The figure shows three views and two pictorial views of one solid part (mm, origin at its lowest corner). Answer the questions. A direction names the side the tool comes from. Coordinates: 2 decimals unless noted, no trailing zeros. Order: outer loops, then holes, each group sorted by start corner. A loop starts at its lowest first (then second) coordinate and runs counter-clockwise, first axis right, second up. Notation, with made-up numbers: (71.25, -31.5) -> (77.25, -31.5) arc R21 ccw to (77.25, -22.5) -> close; hole circle Ø5 at (4.5, 81.25). An arc over 180 degrees is marked (long way). Return JSON: item names as keys, results as strings.
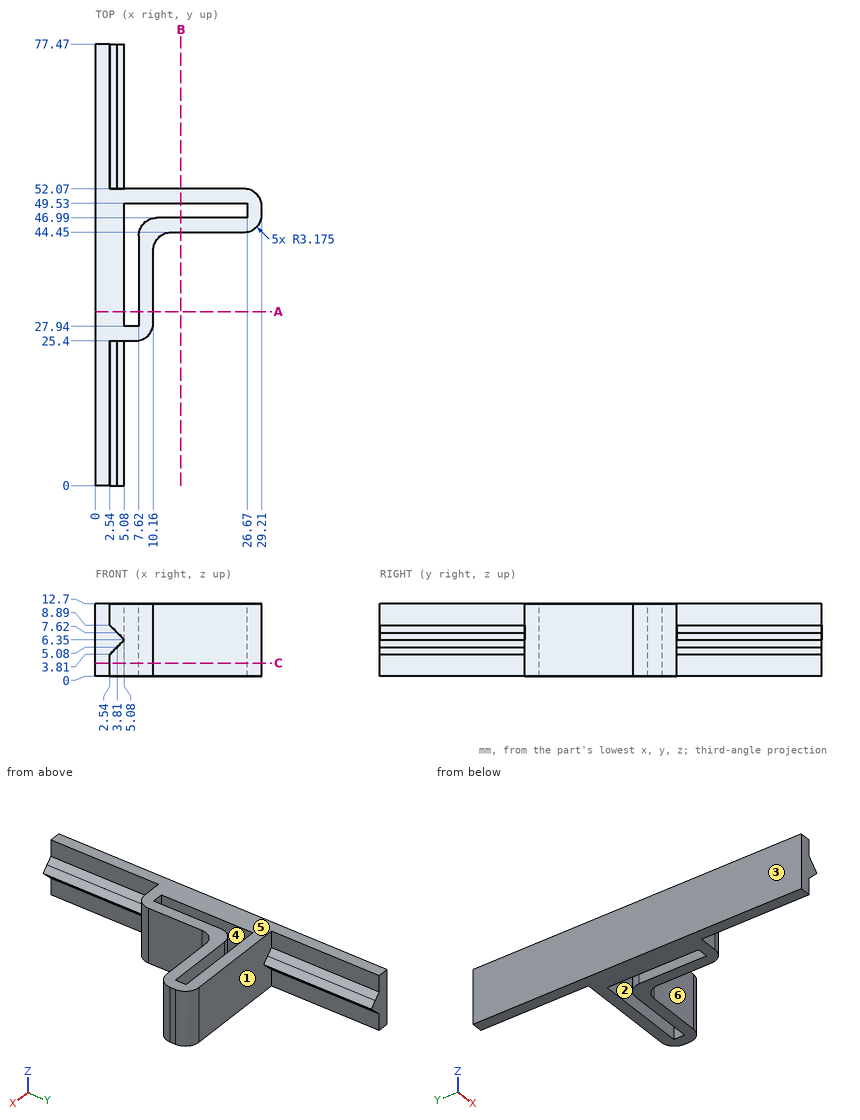
Item 1: Which of the six approach directions +Z, -Z, +X, -X, +Y, -Y give full straight-line access (tool end or side, diameter ignored) to the marked faces 4, 5 and 6?
Answer list:
{"face 4": "+Z, -Z", "face 5": "+Z, +X, -X, +Y, -Y", "face 6": "+Z, -Z, +X, -Y"}
Item 2: Flat-ended cylindrical pins translate along their axes: pin 1 (1.9 mm diameter, centred on y = 59.5, z = 1.5, fed in from +X); pin 2 (1.3 mm diameter, centred on x = 5.5, z = 9, fed in from -Y); pin 3 (5 mm diameter, centred on x = 6, y = 23, fed in from -Z); pin 4 (2 mm diameter, centred on x = 4, y = 66, fed in from +Z). Find the tip coordinate at first contact, or state that the pin passes through.
Answer list:
{"pin 1": "x = 2.54", "pin 2": "y = 25.4", "pin 3": "z = 0", "pin 4": "z = 8.43"}
Item 3: The part is cut by section C-C on z = 2.25. Determine the outline of the cut face in (x, y) (3 decimals), plus the area to 3 significant figures.
Answer list:
{"outline": "(0, 0) -> (2.54, 0) -> (2.54, 25.4) -> (6.985, 25.4) arc R3.175 ccw to (10.16, 28.575) -> (10.16, 41.275) arc R3.175 cw to (13.335, 44.45) -> (26.035, 44.45) arc R3.175 ccw to (29.21, 47.625) -> (29.21, 48.895) arc R3.175 ccw to (26.035, 52.07) -> (2.54, 52.07) -> (2.54, 77.47) -> (0, 77.47) -> close; hole (5.08, 27.94) -> (7.62, 27.94) -> (7.62, 43.815) arc R3.175 cw to (10.795, 46.99) -> (26.67, 46.99) -> (26.67, 49.53) -> (5.08, 49.53) -> close", "area": "435 mm2"}
Item 4: Find the intervals of material crossed by probe 1 along X at (y, z) = (34, 8.5); probe 2 along Y at (x, z) = (24, 1.5); probe 3 along X at (y, z) = (17, 3.5), in increasing order.
Answer list:
{"probe 1": "0 to 5.08, 7.62 to 10.16", "probe 2": "44.45 to 46.99, 49.53 to 52.07", "probe 3": "0 to 2.54"}
Item 5: The part is cut by section A-A on y = 30.5. Determine the outline of the cut face in (x, z), plus the area to 3 significant figures.
Answer list:
{"outline": "(0, 0) -> (5.08, 0) -> (5.08, 12.7) -> (0, 12.7) -> close; (7.62, 0) -> (10.16, 0) -> (10.16, 12.7) -> (7.62, 12.7) -> close", "area": "96.8 mm2"}
Item 6: Determine the mould class of the marked faces 1, 2 and 3 for opening direction Y: pulls with the +Y half, pulls with the -Y half, needs draft (parallel to the pull), parting line crosses it, or undercut.
Answer list:
{"face 1": "pulls with the +Y half", "face 2": "undercut", "face 3": "needs draft"}
Item 7: The part is cut by section B-B on x = 15. Determine the outline of the cut face in (y, z).
Answer list:
{"outline": "(44.45, 0) -> (46.99, 0) -> (46.99, 12.7) -> (44.45, 12.7) -> close; (49.53, 0) -> (52.07, 0) -> (52.07, 12.7) -> (49.53, 12.7) -> close"}
